```python
from build123d import *

# Parameters (mm, degrees)
F0_W      = 65
F0_H      = 1.5
F1_DEPTH  = 15.5
F2_W      = 15
F2_H      = 20
F3_DEPTH  = 20
F4_R      = 4
F5_DEPTH  = 13
F6_R      = 4
F7_DEPTH  = 13
F8_R      = 0.5
F9_DEPTH  = 25.4
F10_R     = 0.5
F11_DEPTH = 25.4


with BuildPart() as f1:
    # F0 (on Front) → F1 (new body, symmetric)
    with BuildSketch(Plane.XZ):
        Rectangle(F0_W, F0_H)
    extrude(amount=F1_DEPTH, both=True)

    # F2 (on face) → F3 (join)
    with BuildSketch(Plane.XY.offset(0.75)):
        with Locations((7, 4.07752)):
            Rectangle(F2_W, F2_H)
    extrude(amount=F3_DEPTH)

    # F4 (on face) → F5 (join)
    with BuildSketch(Plane.XY.offset(0.75)):
        with Locations((-19.5, 10.054756)):
            Circle(F4_R)
    extrude(amount=F5_DEPTH)

    # F6 (on face) → F7 (join)
    with BuildSketch(Plane.XY.offset(0.75)):
        with Locations((22.5, -9.5)):
            Circle(F6_R)
    extrude(amount=F7_DEPTH)

    # F8 (on face) → F9 (cut)
    with BuildSketch(Plane.XY.offset(0.75)):
        with Locations((-30.195765, -13.578762)):
            Circle(F8_R)
    extrude(amount=-F9_DEPTH, mode=Mode.SUBTRACT)

    # F10 (on face) → F11 (cut)
    with BuildSketch(Plane.XY.offset(0.75)):
        with Locations((-18.195813, -13.612677)):
            Circle(F10_R)
    extrude(amount=-F11_DEPTH, mode=Mode.SUBTRACT)


solid = f1.part
```
CAD build for the part. Positions are in the model's coordinates, mm. A direction names the side the tool comes from. Coordinates: 2 decimals unless noted, no trailing zeros. Order: outer loops, then holes, each group sorted by start corner. A loop starts at its lowest first (then second) coordinate and runs counter-clockwise, first axis right, second up.
(1) Saw through at D-D, the plane z = 16.5. Write the cut outline in (x, y).
Solution:
outline: (-0.5, -5.92) - (14.5, -5.92) - (14.5, 14.08) - (-0.5, 14.08) - close
(2) Mould opens along X. For faces 1 (the face through (0, 0, -0.75)), 2 (the face through (-22.448, 12.758, 7.159)), 3 (the face through (32.5, 0, 0)) say: released by +X, released by -X, zero draft, split by the parting line, or undercut.
Solution:
face 1: zero draft
face 2: undercut
face 3: released by +X
(3) Saw through at C-C, the plane z = 12.5. Write the cut outline in (x, y).
Solution:
outline: circle Ø8 at (-19.5, 10.05); (-0.5, -5.92) - (14.5, -5.92) - (14.5, 14.08) - (-0.5, 14.08) - close; circle Ø8 at (22.5, -9.5)
(4) Pin check, flat tips, straight feed: pin 1 Ø1 at (x, z) = (8.5, 7) entering from -Y; pin 2 Ø2.5 at (x, y) = (-21, 11) entering from +Z; pin 3 Ø3 at (y, z) = (-2, 15) entering from -X. Stop position of each tip, or through.
Solution:
pin 1: stops at y = -5.92
pin 2: stops at z = 13.75
pin 3: stops at x = -0.5
(5) Which spindle directions (+Z, -Z, +X, -X, +Y, -Y) get a long thin tool onto all of the face, cutting with end or side? Do faces 4 (the face through (-20, 10, 13.75)), 5 (the face through (-0.5, 4, 11)), 6 (the face through (7, -5.922, 11)), 7 (the face through (19.3, -11.9, 7.2)), 8 (the face through (7, 14.078, 11)). Say none if no direction does.
Solution:
face 4: +Z, -X, +Y, -Y
face 5: +Z, +Y, -Y
face 6: +Z, -X, -Y
face 7: +Z
face 8: +Z, +X, -X, +Y
(6) Saw through at A-A, the plane x = 6.5. Write the cut outline in (y, z).
Solution:
outline: (-15.5, -0.75) - (15.5, -0.75) - (15.5, 0.75) - (14.08, 0.75) - (14.08, 20.75) - (-5.92, 20.75) - (-5.92, 0.75) - (-15.5, 0.75) - close
(7) Drill centre lines: L1, parallel to Z at x = -19, y = -6; L2, parallel to X at y = 11, z = 17.5; L3, parallel to X at y = 13, z = 13.5. Where is each one in solid material? Low to high.
Solution:
L1: z = -0.75 to 0.75
L2: x = -0.5 to 14.5
L3: x = -22.21 to -16.79, -0.5 to 14.5
(8) Saw through at B-B, the plane y = -9.5. Write the cut outline in (x, z), and give its area (4 significant figures).
Solution:
outline: (-32.5, -0.75) - (32.5, -0.75) - (32.5, 0.75) - (26.5, 0.75) - (26.5, 13.75) - (18.5, 13.75) - (18.5, 0.75) - (-32.5, 0.75) - close
area: 201.5 mm2
